Could you check a few things on this model? Use its own coordinates, in mm. A direction names the side the tool comes from. Round coordinates to 2 decimals unless told otherwise and drop trailing zeros. Loops run counter-clockwise (first coordinate to the right, second up) from the corner with the lowest first, then second, coordinate; pieces in that order, holes last. Notation, with made-up numbers: M 52,31 L 87,31 A17 cw 87,41 Z; hole C 46.5,17 d2. An arc over 180 degrees is marked long. Return JSON: item names as keys, results as strings. Group by question number.
```python
from build123d import *

# Parameters (mm, degrees)
F0_W      = 40
F0_H      = 48
F1_DEPTH  = 25
F3_W      = 42
F3_H      = 25
F4_DEPTH  = 37
F2_W      = 3
F2_H      = 25
F5_DEPTH  = 10
F6_W      = 3
F6_H      = 25
F7_DEPTH  = 10
F8_R      = 5
F11_DEPTH = 25


with BuildPart() as f1:
    # F0 (on Top) → F1 (new body)
    with BuildSketch(Plane.XY):
        Rectangle(F0_W, F0_H)
    extrude(amount=F1_DEPTH)

    # F3 (on face) → F4 (cut)
    with BuildSketch(Plane.YZ.offset(20)):
        with Locations((0, 12.5)):
            Rectangle(F3_W, F3_H)
    extrude(amount=-F4_DEPTH, mode=Mode.SUBTRACT)

    # F2 (on face) → F5 (join)
    with BuildSketch(Plane.XZ.offset(24)):
        with Locations((-18.5, 12.5)):
            Rectangle(F2_W, F2_H)
    extrude(amount=F5_DEPTH)

    # F6 (on face) → F7 (join)
    with BuildSketch(Plane(origin=(0, 24, 0), x_dir=(-1, 0, 0), z_dir=(0, 1, 0))):
        with Locations((18.5, 12.5)):
            Rectangle(F6_W, F6_H)
    extrude(amount=F7_DEPTH)

    # F8
    f8_edges = [f1.edges().sort_by_distance(p)[0] for p in [
        (-18.5, 34, 0),
        (-18.5, 34, 25),
        (-18.5, -34, 0),
        (-18.5, -34, 25),
    ]]
    fillet(f8_edges, radius=F8_R)

    # F10 (on face) + F9 (on face) → F11 (cut)
    with BuildSketch(Plane.YZ.offset(-17)):
        with BuildLine():
            ThreePointArc((29, 15.5), (26, 12.5), (29, 9.5))
            Line((29, 9.5), (29, 15.5))
        make_face()
        with BuildLine():
            Line((29, 15.5), (29, 9.5))
            ThreePointArc((29, 9.5), (31.1213203436, 10.3786796564), (32, 12.5))
            ThreePointArc((32, 12.5), (31.1213203436, 14.6213203436), (29, 15.5))
        make_face()
    with BuildSketch(Plane.YZ.offset(-17)):
        with BuildLine():
            ThreePointArc((-29, 15.5), (-32, 12.5), (-29, 9.5))
            Line((-29, 9.5), (-29, 15.5))
        make_face()
        with BuildLine():
            Line((-29, 15.5), (-29, 9.5))
            ThreePointArc((-29, 9.5), (-26.8786796564, 10.3786796564), (-26, 12.5))
            ThreePointArc((-26, 12.5), (-26.8786796564, 14.6213203436), (-29, 15.5))
        make_face()
    extrude(amount=-F11_DEPTH, mode=Mode.SUBTRACT)


solid = f1.part
```
1. We'd pull the mould along Y, two halves only. Please class faces 4 (the face through (-18, -33, 23)), 5 (the face through (2, 21, 12)), 6 (the face through (20, 22, 12)): +Y half, -Y half, draft (parallel to the pull), parting line (faces both ways), or undercut.
2. If we section it at B-B, the plane z = 8.5: Please give me the cut outline in (x, y).
3. If we section it at D-D, the plane y = 14: Please give me the cut outline in (x, z).
4. On a 3-axis mill with a long thin cutter (end or side, diameter ignored), from which of +Z, -Z, +X, -X, +Y, -Y can I reach the whole of each face in a straight line? I mean faces 1 (the face through (-17, 0, 13)), 2 (the face through (-17, -27.8, 9.5)), 3 (the face through (-17, 27.8, 9.5)). Say none if no direction works.
5. I need wall thicknesses on probe 1 along Y at (x, z) = (-9, 23.75); probe 2 along Y at (x, z) = (-17.5, 13); probe 3 along X at (y, z) = (14.5, 7). Which ranges of each line are inside material? Lowest first, please.
6. If we section it at C-C, the plane y = 30: Please give me the cut outline in (x, z).
7. If we section it at A-A, the plane x = 2.5: Please give me the cut outline in (y, z).
8. I'm going to push flat-ended pins straight in: pin 1 Ø4 at (x, z) = (-2.5, 18) entering from +Y; pin 2 Ø5 at (y, z) = (-17, 3) entering from +X; pin 3 Ø12 at (x, y) = (6, 18) entering from +Z; pin 4 Ø7.5 at (x, z) = (-0.5, 7.5) entering from -Y. Where does each tip first touch, or does it pass through?
Geometry results:
{
 "1": {"face 4": "-Y half", "face 5": "undercut", "face 6": "draft"},
 "2": {"outline": "M -20,-34 L -17,-34 L -17,-24 L 20,-24 L 20,-21 L -17,-21 L -17,21 L 20,21 L 20,24 L -17,24 L -17,34 L -20,34 Z"},
 "3": {"outline": "M -20,0 L -17,0 L -17,25 L -20,25 Z"},
 "4": {"face 1": "+Z, -Z, +X", "face 2": "+Z, -Z, +X, -Y", "face 3": "+Z, -Z, +X, +Y"},
 "5": {"probe 1": "-24 to -21, 21 to 24", "probe 2": "-34 to -31.96, -26.04 to 26.04, 31.96 to 34", "probe 3": "-20 to -17"},
 "6": {"outline": "M -20,0.1 L -17,0.1 L -17,9.67 L -20,9.67 Z; M -20,15.33 L -17,15.33 L -17,24.9 L -20,24.9 Z"},
 "7": {"outline": "M -24,0 L -21,0 L -21,25 L -24,25 Z; M 21,0 L 24,0 L 24,25 L 21,25 Z"},
 "8": {"pin 1": "y = 24", "pin 2": "x = -17", "pin 3": "z = 25", "pin 4": "y = -24"}
}
